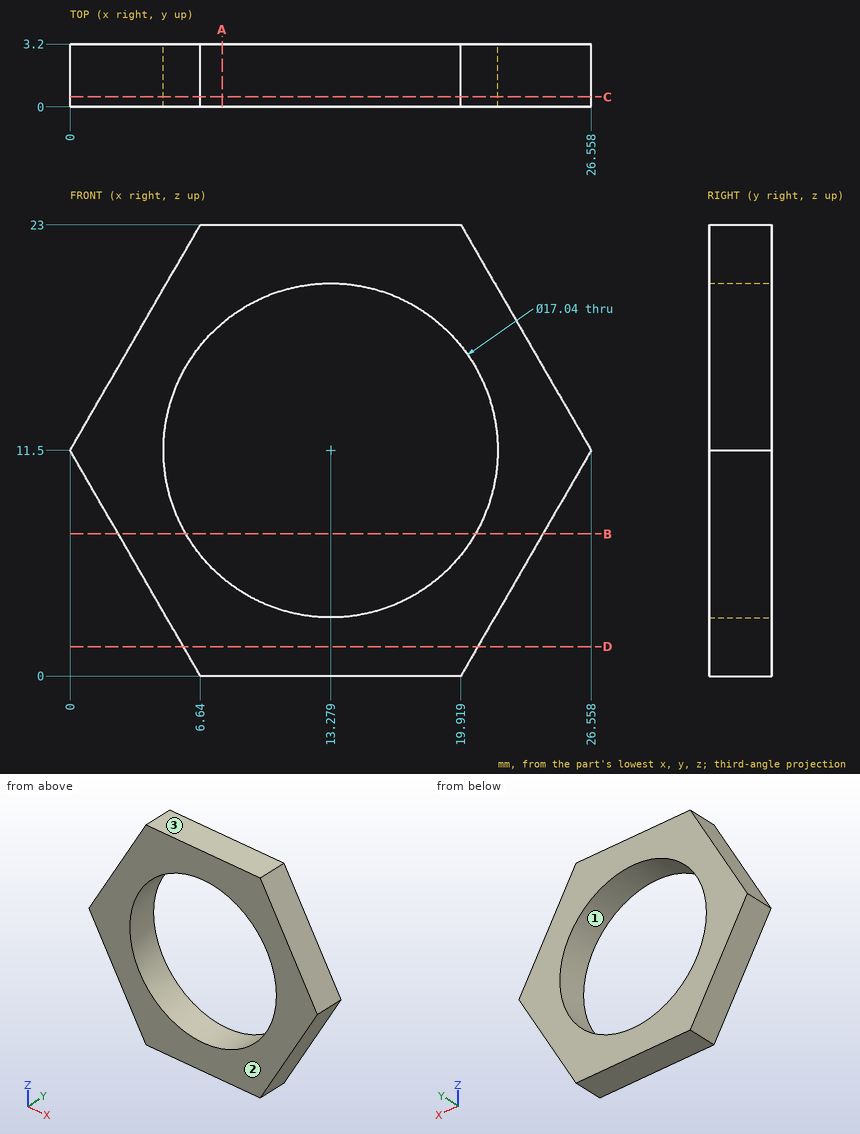
Source: three-view drawing plus pictorial views. Frame: mm from the lowest corner of the part. Coordinates: 2 decimals unless noted, no trailing zeros. Loops run counter-clockwise (first coordinate to the right, second up) from the corner with the lowest first, then second, coordinate; pieces in that order, holes last. Notation, with made-up numbers: (14, -19.5) -> (41, -19.5) arc R24 ccw to (41, 3.5) -> close; hole circle Ø3 at (-25, 79). An arc over 180 degrees is marked (long way). Write each question's results on one line, items separated by ' | '. Start each with the question number.
Q1. Pin query (flat end, axial travel): pin 1 (1 mm diameter, centred on y = 1.5, z = 18, fed in from +X) (1 decimal); pin 2 (1 mm diameter, centred on y = 2.5, z = 9, fed in from -X) (1 decimal). Return the tip coordinate at first contact, or that it passes through.
Q2. Section C-C, the plane y = 0.5. Return the cut outline in (x, z).
Q3. Ray query, line 1 (Z direction, x = 13, y = 0.3) (1 decimal); line 2 (X direction, y = 0.5, z = 18.5) (1 decimal); line 3 (Z direction, x = 8.5, y = 0.9) (1 decimal). Return the intervals inside material, ascending. Write a range as from..to.
Q4. Section D-D, the plane z = 1.5. Return the cut outline in (x, y) (1 decimal).
Q5. Section A-A, the plane x = 7.75. Return the cut outline in (y, z), plus the area to 3 significant figures.
Q6. Section B-B, the plane z = 7.25. Return the cut outline in (x, y) (1 decimal), plus the area to 3 significant figures.
Q7. Pull-direction query (Z, two-part tool) for the marked faces 1, 2 and 3; classes: released by +Z, released by -Z, zero draft, split by the parting line, or undercut.
Found:
1) pin 1: x = 23.1 | pin 2: x = 1.2
2) outline: (0, 11.5) -> (6.64, 0) -> (19.92, 0) -> (26.56, 11.5) -> (19.92, 23) -> (6.64, 23) -> close; hole circle Ø17.04 at (13.28, 11.5)
3) line 1: 0..3, 20..23 | line 2: 4..8.4, 18.1..22.5 | line 3: 0..4.4, 18.6..23
4) outline: (5.8, 0) -> (20.8, 0) -> (20.8, 3.2) -> (5.8, 3.2) -> close
5) outline: (0, 0) -> (3.2, 0) -> (3.2, 5.02) -> (0, 5.02) -> close; (0, 17.98) -> (3.2, 17.98) -> (3.2, 23) -> (0, 23) -> close | area: 32.1 mm2
6) outline: (2.5, 0) -> (5.9, 0) -> (5.9, 3.2) -> (2.5, 3.2) -> close; (20.7, 0) -> (24.1, 0) -> (24.1, 3.2) -> (20.7, 3.2) -> close | area: 22.0 mm2
7) face 1: undercut | face 2: zero draft | face 3: released by +Z
